```python
from build123d import *

# Parameters (mm, degrees)
CYLINDER119_R             = 5
CYLINDER119_DEPTH         = 7
CYLINDER118_R             = 8.55
CYLINDER118_DEPTH         = 7
CHAMFER005_SIZE           = 2
CYLINDER117_R             = 10
CYLINDER117_DEPTH         = 3
CHAMFER006_SIZE           = 1.54
FILLET006_R               = 1
FILLET006_PLACEMENT_ANGLE = 90


with BuildPart() as cylinder119:
    # Cylinder119 → Cylinder119 (new body)
    with BuildSketch(Plane.XY.offset(5)):
        Circle(CYLINDER119_R)
    extrude(amount=CYLINDER119_DEPTH)


with BuildPart() as fusion112:
    # Cylinder118 → Cylinder118 (new body)
    with BuildSketch(Plane.XY.offset(7)):
        Circle(CYLINDER118_R)
    extrude(amount=CYLINDER118_DEPTH)

    # Chamfer005
    chamfer005_edges = [fusion112.edges().sort_by_distance(p)[0] for p in [
        (-8.55, 0, 7),
    ]]
    chamfer(chamfer005_edges, length=CHAMFER005_SIZE)

    # Fusion112: union Cylinder119
    add(cylinder119.part)


with BuildPart() as cylinder117:
    # Cylinder117 → Cylinder117 (new body)
    with BuildSketch(Plane.XY.offset(11)):
        Circle(CYLINDER117_R)
    extrude(amount=CYLINDER117_DEPTH)


with BuildPart() as hub_wide_cap_left:
    # Cone → Cone (revolve)
    with BuildSketch(Plane(origin=(0, 0, 3), x_dir=(1, 0, 0), z_dir=(0, -1, 0))):
        Polygon((0, 0), (6, 0), (10, 8), (0, 8), align=None)
    revolve(axis=Axis((0, 0, 3), (0, 0, 1)))

    # Fusion111: union Cylinder117
    add(cylinder117.part)

    # Cut039: cut Fusion112
    add(fusion112.part, mode=Mode.SUBTRACT)

    # Chamfer006
    chamfer006_edges = [hub_wide_cap_left.edges().sort_by_distance(p)[0] for p in [
        (-5, 0, 7),
    ]]
    chamfer(chamfer006_edges, length=CHAMFER006_SIZE)

    # Fillet006
    fillet006_edges = [hub_wide_cap_left.edges().sort_by_distance(p)[0] for p in [
        (-10, 0, 11),
        (-6, 0, 3),
    ]]
    fillet(fillet006_edges, radius=FILLET006_R)


with BuildPart() as hub_wide_cap_left_1:
    # Fillet006 placement: moved
    add(hub_wide_cap_left.part.moved(Location((0, -88, 0))).rotate(Axis((0, -88, 0), (-1, 0, 0)), FILLET006_PLACEMENT_ANGLE))


solid = hub_wide_cap_left_1.part
```
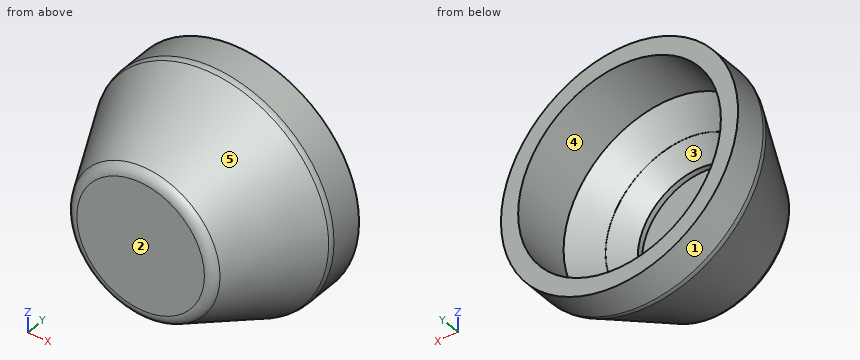
Design review of the part built by this model. Coordinates are the model's own, in mm. Face numbers are marked on the shaded views. A direction names the side the tool comes from. Round coordinates to 2 decimals unless told otherwise and drop trailing zeros. Order: outer loops, then holes, each group sorted by start corner. A loop starts at its lowest first (then second) coordinate and runs counter-clockwise, first axis right, second up. Notation, with made-up numbers: (46.5, 37.25) - (58.5, 37.25) arc R16 ccw to (58.5, 66.25) - close; hole circle Ø2 at (81, 60.5). An arc over 180 degrees is marked (long way). Return JSON: item names as keys, results as strings.
Q1. For pin 1 Ø5 at (y, z) = (-80, 3.5) entering from +X; pin 2 Ø3 at (x, z) = (-1.5, -2.5) entering from +Y; pin 3 Ø1 at (x, y) = (-3.5, -79.5) entering from +Z, all flat-tipped, find the tip position at first contact; note any pin that passes through.
Computed values:
{"pin 1": "stops at x = 9.32", "pin 2": "stops at y = -83", "pin 3": "stops at z = 8.36"}
Q2. Consider section A-A on y = -82. Write out the cut boundary in (x, z), plus the area to 3 significant figures.
Computed values:
{"outline": "circle Ø15 at (0, 0); hole circle Ø11.08 at (0, 0)", "area": "80.3 mm2"}
Q3. The part is to be moulded in two halves that separate along X. For the marked faces 1, 2 and 3, say which applies: pulls with the +X half, pulls with the -X half, needs draft (parallel to the pull), parting line crosses it, or undercut.
Computed values:
{"face 1": "parting line crosses it", "face 2": "needs draft", "face 3": "undercut"}
Q4. Wall thickness on L1, parallel to Z at x = 0, y = -76.4; L2, parallel to X at y = -78, z = -3.5; L3, parallel to Z at x = 1.25, y = -80: over which ranges is each line inside the solid? List them lowest first. Write a range as [from, to].
Computed values:
{"L1": "z = [-10, -8.55], [8.55, 10]", "L2": "x = [-8.83, -7.8], [7.8, 8.83]", "L3": "z = [-8.41, -7.45], [7.45, 8.41]"}
Q5. Machinability: for the marked faces 4 and 5, which of the approach directions +Z, -Z, +X, -X, +Y, -Y give a long, thin tool a straight path to every point of the face, cutting with its end or side? Answer none if there is none.
Computed values:
{"face 4": "+Y", "face 5": "-Y"}
Q6. Consider section B-B on y = -79.5. Write out the cut boundary in (x, z), plus the area to 3 significant figures.
Computed values:
{"outline": "circle Ø17.5 at (0, 0); hole circle Ø16.1 at (0, 0)", "area": "36.9 mm2"}
